Geometry check sheet. Reference: the model listing, model coordinates, mm. Coordinates: 2 decimals unless noted, no trailing zeros. Loops run counter-clockwise (first coordinate to the right, second up) from the corner with the lowest first, then second, coordinate; pieces in that order, holes last.
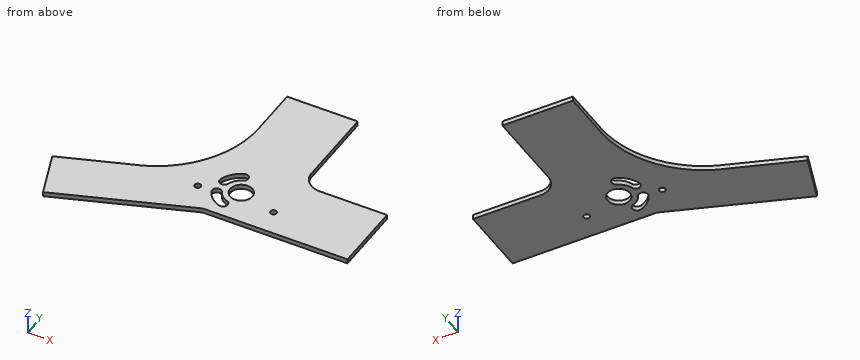
Autodesk Inventor part; units mm, degrees
ref_plane "YZ Plane" through (0, 0, 0) normal (1, 0, 0) x (0, 1, 0)
ref_plane "XZ Plane" through (0, 0, 0) normal (0, 1, 0) x (-1, 0, 0)
ref_plane "XY Plane" through (0, 0, 0) normal (0, 0, 1) x (1, 0, 0)
ref_plane "РабПлоскость5" through (0, 0, -194) normal (0, 0, 1) x (1, 0, 0)
sketch "Эскиз4" plane through (0, 0, -194) normal (0, 0, 1) x (1, 0, 0)
  line L0 (-7.3772, -14.0792) -> (50, -14.0792)
  line L1 (-60, -33.2323) -> (-7.3772, -14.0792)
  line L2 (-66.8404, -14.4385) -> (-60, -33.2323)
  line L3 (-40.9989, -5.0329) -> (-66.8404, -14.4385)
  arc A0 (-40.9989, -5.0329) -> (-12, 33.9208) centre (-52.4998, 33.7998) ccw
  line L4 (-12, 53.9208) -> (-12, 33.9208)
  line L5 (16, 53.9208) -> (-12, 53.9208)
  line L6 (16, 22.4208) -> (16, 53.9208)
  arc A1 (16, 22.4208) -> (23, 13.9208) centre (23.4314, 21.4084) ccw
  line L7 (50, 13.9208) -> (23, 13.9208)
  line L8 (50, -14.0792) -> (50, 13.9208)
  point P0 (0, 0)
extrude "Выдавливание4" add sketch "Эскиз4" along normal blind 1.8
sketch "Эскиз5" plane through (0, 0, -192.2) normal (0, 0, 1) x (1, 0, 0)
  circle A0 centre (0, 0) radius 4.4
  circle A1 centre (0, 0) radius 12
  circle A2 centre (15, -4) radius 1.2
  line L0 (0, 0) -> (0, -30) construction
  circle A3 centre (-15, -4) radius 1.2
  arc A4 (-3.4374, 7.8273) -> (-8.1316, 2.6381) centre (0, 0) ccw construction
  arc A5 (-4.1781, 9.5141) -> (-9.8839, 3.2066) centre (0, 0) ccw
  arc A6 (-2.6966, 6.1406) -> (-6.3793, 2.0696) centre (0, 0) ccw
  arc A7 (-2.6966, 6.1406) -> (-4.1781, 9.5141) centre (-3.4374, 7.8273) ccw
  arc A8 (-9.8839, 3.2066) -> (-6.3793, 2.0696) centre (-8.1316, 2.6381) ccw
  arc A9 (-7.7059, -3.7016) -> (-2.6966, -8.1124) centre (0, 0) ccw construction
  arc A10 (-9.3665, -4.4992) -> (-3.2777, -9.8605) centre (0, 0) ccw
  arc A11 (-6.0453, -2.9039) -> (-2.1155, -6.3642) centre (0, 0) ccw
  arc A12 (-6.0453, -2.9039) -> (-9.3665, -4.4992) centre (-7.7059, -3.7016) ccw
  arc A13 (-3.2777, -9.8605) -> (-2.1155, -6.3642) centre (-2.6966, -8.1124) ccw
  dimension "d42" = 8.8
  dimension "d43" = 24
  dimension "d44" = 2.4
  dimension "d46" = 30
  dimension "d47" = 15
  dimension "d48" = 4
extrude "Выдавливание5" cut sketch "Эскиз5" against normal blind 30 contours A0 | A2 | A3 | A7 A6 A8 A5 | A12 A11 A13 A10
equation "\"d49\" = d46"
properties part number "Обхват головы"
(1) Sectioned sample at C-C on y = -27.5. Record the cut outline in (x, z), and give its area (3 significant figures).
Findings:
outline: (-62.09, -194) - (-44.25, -194) - (-44.25, -192.2) - (-62.09, -192.2) - close
area: 32.1 mm2
(2) Sectioned sample at D-D on x = -38. Record the cut outline in (y, z), and give its area (3 significant figures).
Findings:
outline: (-25.22, -194) - (-4.02, -194) - (-4.02, -192.2) - (-25.22, -192.2) - close
area: 38.2 mm2
(3) Scan lines: L1, parallel to Y at x = 0, z = -192.95; L2, parallel to X at y = 1, z = -192.8; L3, parallel to Y at x = 15, z = -193.5. Record each from-to range of solid material in increasing order.
Findings:
L1: y = -14.08 to -4.4, 4.4 to 53.92
L2: x = -28.74 to -8.97, -7.29 to -4.28, 4.28 to 50
L3: y = -14.08 to -5.2, -2.8 to 53.92
(4) Sectioned sample at B-B on x = -15. Record the cut outline in (y, z), and give its area (3 significant figures).
Findings:
outline: (-16.85, -194) - (-5.2, -194) - (-5.2, -192.2) - (-16.85, -192.2) - close; (-2.8, -194) - (18.5, -194) - (18.5, -192.2) - (-2.8, -192.2) - close
area: 59.3 mm2
(5) Sectioned sample at A-A on z = -192.5. Record the cut outline in (x, y), and give its area (3 significant figures).
Findings:
outline: (-66.84, -14.44) - (-60, -33.23) - (-7.38, -14.08) - (50, -14.08) - (50, 13.92) - (23, 13.92) arc R7.5 cw to (16, 22.42) - (16, 53.92) - (-12, 53.92) - (-12, 33.92) arc R40.5 cw to (-41, -5.03) - close; hole circle Ø2.4 at (-15, -4); hole (-9.88, 3.21) arc R1.84 ccw to (-6.38, 2.07) arc R6.71 cw to (-2.7, 6.14) arc R1.84 ccw to (-4.18, 9.51) arc R10.39 ccw to start; hole (-9.37, -4.5) arc R10.39 ccw to (-3.28, -9.86) arc R1.84 ccw to (-2.12, -6.36) arc R6.71 cw to (-6.05, -2.9) arc R1.84 ccw to start; hole circle Ø8.8 at (0, 0); hole circle Ø2.4 at (15, -4)
area: 3,970 mm2
(6) Gauge pin test, flat ends, axial feed: pin 1 Ø0.9 at (x, z) = (25.5, -193) entering from -Y; pin 2 Ø1 at (x, z) = (-53, -193.5) entering from -Y; pin 3 Ø0.5 at (y, z) = (42.5, -193) entering from +X. Record the tip position at first contact, or that the pin passes through.
Findings:
pin 1: stops at y = -14.08
pin 2: stops at y = -30.87
pin 3: stops at x = 16
